Here's the drawing with two shaded views (mm, measured from the low corner). I have some questions. Give positions to 0.01 mm unless a question says otherwise; leave off trailing zeros. Write each loop counter-clockwise with the first axis right and the second up, starting at its lowest first coordinate (ties: lowest second). Pieces come first, ordered by that corner, then holes.
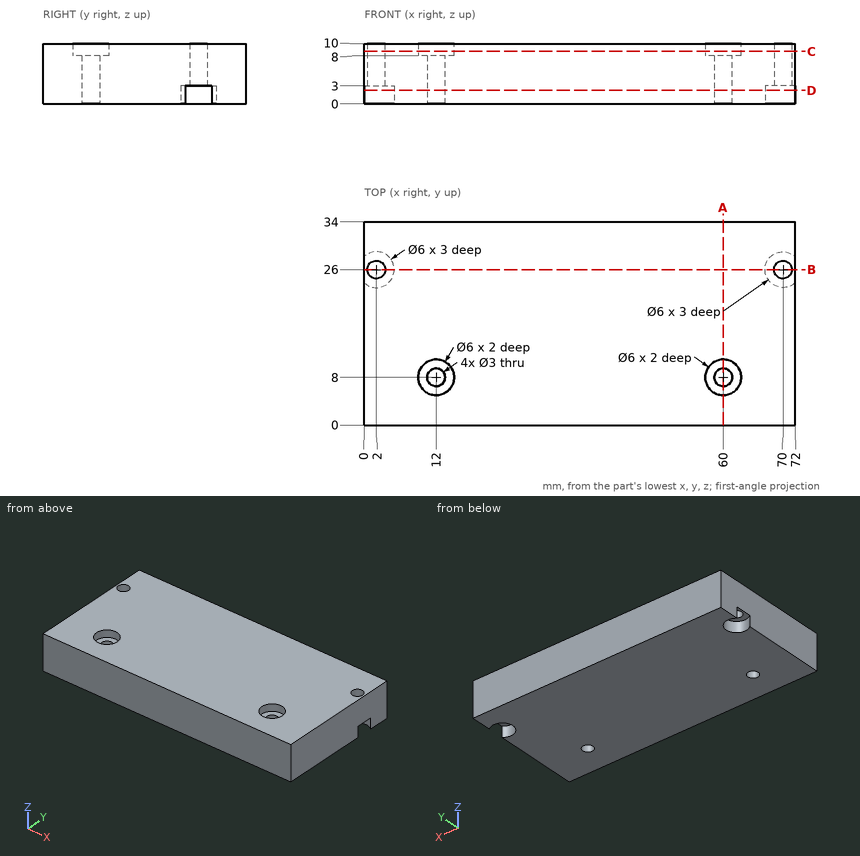
1) Suppose I cut it at A-A on x = 60. Write out the boundary of the cut face in (y, z), plus the area to 3 significant figures.
Values follow:
outline: (0, 0) - (6.5, 0) - (6.5, 8) - (5, 8) - (5, 10) - (0, 10) - close; (9.5, 0) - (34, 0) - (34, 10) - (11, 10) - (11, 8) - (9.5, 8) - close
area: 304 mm2
2) Suppose I cut it at C-C on z = 8.75. Write out the boundary of the cut face in (x, y).
Values follow:
outline: (0, 0) - (72, 0) - (72, 34) - (0, 34) - close; hole circle Ø3 at (2, 26); hole circle Ø6 at (12, 8); hole circle Ø6 at (60, 8); hole circle Ø3 at (70, 26)
3) Please list where these lines run through material, in increasing order: L1, parallel to X at y = 8, z = 3.25; L2, parallel to X at y = 26, z = 7.25; L3, parallel to Y at x = 60, z = 3.5.
Values follow:
L1: x = 0 to 10.5, 13.5 to 58.5, 61.5 to 72
L2: x = 0 to 0.5, 3.5 to 68.5, 71.5 to 72
L3: y = 0 to 6.5, 9.5 to 34
4) Suppose I cut it at B-B on y = 26. Write out the boundary of the cut face in (x, z), plus the area to 3 significant figures.
Values follow:
outline: (0, 3) - (0.5, 3) - (0.5, 10) - (0, 10) - close; (3.5, 3) - (5, 3) - (5, 0) - (67, 0) - (67, 3) - (68.5, 3) - (68.5, 10) - (3.5, 10) - close; (71.5, 3) - (72, 3) - (72, 10) - (71.5, 10) - close
area: 648 mm2
5) For pin 1 Ø5 at (x, y) = (60, 8) entering from +Z; pin 2 Ø1.8 at (x, y) = (70, 26) entering from -Z; pin 3 Ø5 at (x, y) = (2, 26) entering from -Z, each with a flat end and sliding along its axis, tell me the tip position at first contact or that it passes through.
Values follow:
pin 1: stops at z = 8
pin 2: passes through
pin 3: stops at z = 3
6) Suppose I cut it at D-D on z = 2.25. Write out the boundary of the cut face in (x, y).
Values follow:
outline: (0, 0) - (72, 0) - (72, 23.76) arc R3 cw (long way) to (72, 28.24) - (72, 34) - (0, 34) - (0, 28.24) arc R3 cw (long way) to (0, 23.76) - close; hole circle Ø3 at (12, 8); hole circle Ø3 at (60, 8)
